Could you check a few things on this drawing? It's one solid part, dimensions in mm from its lowest x, y, z. A direction names the side the tool comes from. Coordinates: 2 decimals unless noted, no trailing zeros. Order: outer loops, then holes, each group sorted by start corner. A loop starts at its lowest first (then second) coordinate and runs counter-clockwise, first axis right, second up. Notation, with made-up numbers: (15, 40.5) -> (37, 40.5) arc R23 cw to (37, 51.5) -> close; hole circle Ø2 at (37.25, 54). An arc over 180 degrees is marked (long way). Answer as CSV lines item,"result".
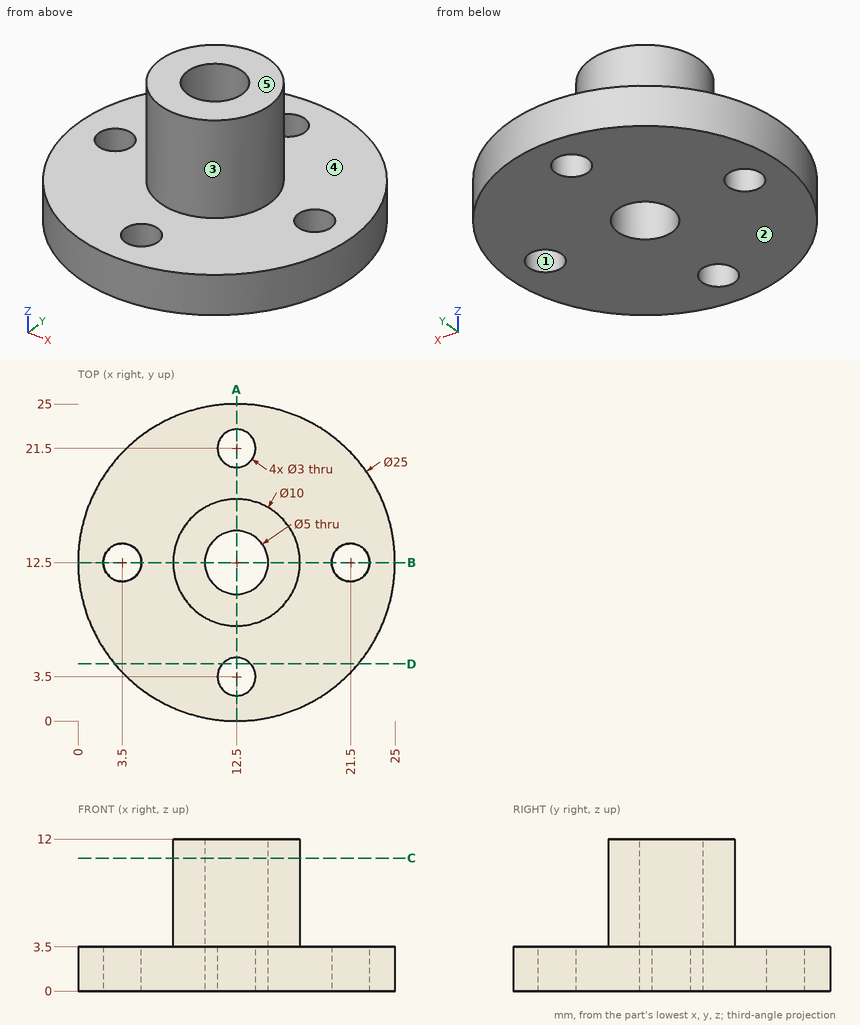
Q1. Imagine slicing it at A-A (x = 12.5). List the corners of the cut face in (y, z) for me.
Solution:
outline,"(0, 0) -> (2, 0) -> (2, 3.5) -> (0, 3.5) -> close; (5, 0) -> (10, 0) -> (10, 12) -> (7.5, 12) -> (7.5, 3.5) -> (5, 3.5) -> close; (15, 0) -> (20, 0) -> (20, 3.5) -> (17.5, 3.5) -> (17.5, 12) -> (15, 12) -> close; (23, 0) -> (25, 0) -> (25, 3.5) -> (23, 3.5) -> close"
Q2. For P1, Ø1.8, axis at x = 3.5, y = 12.5, coming from the -Z side; P2, Ø5, axis at y = 19, z = 10, coming from the +X side; P3, Ø3, axis at y = 6, z = 4, coming from the -X side; P4, Ø4, axis at y = 16.5, z = 2.5, coming from the +X side, each with a flat end and sliding along its axis, tell me the tip position at first contact or that it passes through.
Solution:
P1,"through"
P2,"x = 15.5"
P3,"x = 1.08"
P4,"x = 24.84"
Q3. Imagine slicing it at D-D (y = 4.5). List the corners of the cut face in (x, z) for me.
Solution:
outline,"(2.9, 0) -> (11.38, 0) -> (11.38, 3.5) -> (2.9, 3.5) -> close; (13.62, 0) -> (22.1, 0) -> (22.1, 3.5) -> (13.62, 3.5) -> close"
Q4. If I drill on line 1 (Y direction, x = 12.5, z = 2.5); line 2 (Y direction, x = 12.5, z = 7.75); line 3 (Z direction, x = 6.75, y = 15), over which ranges is the centre line in solid material (lowest first)?
Solution:
line 1,"0 to 2, 5 to 10, 15 to 20, 23 to 25"
line 2,"7.5 to 10, 15 to 17.5"
line 3,"0 to 3.5"
Q5. We'd pull the mould along X, two halves only. Please class the marked faces 1, 2 and 3: pulls with the +X half, pulls with the -X half, needs draft (parallel to the pull), parting line crosses it, or undercut.
Solution:
face 1,"undercut"
face 2,"needs draft"
face 3,"parting line crosses it"
Q6. Which directions (+Z, -Z, +X, -X, +Y, -Y) give clear straight access to the entire face, cutting with the end or side of a thin tool? Please do the marked faces 4 and 5.
Solution:
face 4,"+Z"
face 5,"+Z, +X, -X, +Y, -Y"
Q7. Imagine slicing it at C-C (z = 10.5). List the corners of the cut face in (x, y) for me.
Solution:
outline,"circle Ø10 at (12.5, 12.5); hole circle Ø5 at (12.5, 12.5)"
